from build123d import *

# Parameters (mm, degrees)
EXTRUSION1_DEPTH             = 14
ESQUISSE2_R                  = 3.375
ENL_V_MAT_EXTRU_1_DEPTH      = 11
ENL_V_MAT_EXTRU_2_DEPTH      = 9.5000001
ENL_V_MAT_EXTRU_2_DEPTH_BACK = 9.5000001


with BuildPart() as part:
    # Esquisse1 → Extrusion1 (new body, symmetric)
    with BuildSketch(Plane.XY):
        with BuildLine():
            Line((-8.5, -4.242640687), (-8.5, -3.5))
            ThreePointArc((-8.5, -3.5), (-7.328427125, -0.671572875), (-4.5, 0.5))
            Line((-4.5, 0.5), (4.5, 0.5))
            ThreePointArc((4.5, 0.5), (7.328427125, -0.671572875), (8.5, -3.5))
            Line((8.5, -3.5), (8.5, -4.242640687))
            ThreePointArc((8.5, -4.242640687), (0, -9.5), (-8.5, -4.242640687))
        make_face()
    extrude(amount=EXTRUSION1_DEPTH, both=True)

    # Esquisse2 → Enlèv. mat.-Extru.1 (cut, through all)
    with BuildSketch(Plane(origin=(0, 0.5, 0), x_dir=(-1, 0, 0), z_dir=(0, 1, 0))):
        Circle(ESQUISSE2_R)
    extrude(amount=-ENL_V_MAT_EXTRU_1_DEPTH, mode=Mode.SUBTRACT)

    # Esquisse3 → Enlèv. mat.-Extru.2 (cut, two sides)
    with BuildSketch(Plane(origin=(0, 0, 0), x_dir=(0, 0, -1), z_dir=(1, 0, 0))) as enl_v_mat_extru_2_sk:
        Polygon((14, -9.5), (14, -4.242640687), (9, -9.5), align=None)
        Polygon((-14, -9.5), (-14, -4.242640687), (-9, -9.5), align=None)
    extrude(amount=ENL_V_MAT_EXTRU_2_DEPTH, mode=Mode.SUBTRACT)
    extrude(enl_v_mat_extru_2_sk.sketch, amount=-ENL_V_MAT_EXTRU_2_DEPTH_BACK, mode=Mode.SUBTRACT)


solid = part.part
Read the model definition and answer for the solid it produces. Units are mm, in the model's axes. Coordinates: 2 decimals unless noted, no trailing zeros. Loops run counter-clockwise (first coordinate to the right, second up) from the corner with the lowest first, then second, coordinate; pieces in that order, holes last.
Q1. Consider probe 1 along Z at (x, y) = (0, -2) (3 decimals); probe 2 along X at (y, z) = (-4.25, 0) (3 decimals); probe 3 along Z at (x, y) = (1, -1.5). Determine where each line is inside the solid, lowest interval first.
Q2. The part is cut by section A-A on x = 0. Write down the section's boundary in (y, z) (3 decimals), and give its area (3 significant figures).
Q3. The part is cut by section B-B on z = 0. Write down the section's boundary in (x, y) (3 decimals), and give its area (3 significant figures).
Q4. Each of these flat-tipped pins is pushed along its axis until it touches: pin 1 Ø1 at (y, z) = (-7, 0.5) entering from -X; pin 2 Ø5 at (y, z) = (-8, 4) entering from -X; pin 3 Ø8 at (x, z) = (-6, 0) entering from -Y. Where does it stop, or does it pass through?
Q5. The part is cut by section D-D on z = 9.75. Write down the section's boundary in (x, y).
Q6. The part is cut by section C-C on y = -0.5. Write down the section's boundary in (x, z) (3 decimals).
Q7. The mould has two halves that part along X. Classify faces 1 (the face through (7.297, -0.641, 0.196)), 2 (the face through (0, -2, -14)), 3 (the face through (0.7, -4.4, -3.3)): +X half, -X half, draft (parallel to the pull), parting line (faces both ways), or undercut.
Results below:
1. probe 1: z = -14 to -3.375, 3.375 to 14
1. probe 2: x = -8.496 to -3.375, 3.375 to 8.496
1. probe 3: z = -14 to -3.22, 3.22 to 14
2. outline: (-9.5, -9) - (-4.243, -14) - (0.5, -14) - (0.5, -3.375) - (-9.5, -3.375) - close; (-9.5, 3.375) - (0.5, 3.375) - (0.5, 14) - (-4.243, 14) - (-9.5, 9) - close
2. area: 186 mm2
3. outline: (-8.5, -4.243) arc R9.5 ccw to (-3.375, -8.88) - (-3.375, 0.5) - (-4.5, 0.5) arc R4 ccw to (-8.5, -3.5) - close; (3.375, -8.88) arc R9.5 ccw to (8.5, -4.243) - (8.5, -3.5) arc R4 ccw to (4.5, 0.5) - (3.375, 0.5) - close
3. area: 71.6 mm2
4. pin 1: stops at x = -6.93
4. pin 2: stops at x = -7.75
4. pin 3: stops at y = -9.13
5. outline: (-8.5, -4.24) arc R9.5 ccw to (-3.79, -8.71) - (3.79, -8.71) arc R9.5 ccw to (8.5, -4.24) - (8.5, -3.5) arc R4 ccw to (4.5, 0.5) - (-4.5, 0.5) arc R4 ccw to (-8.5, -3.5) - close
6. outline: (-7.146, -14) - (7.146, -14) - (7.146, 14) - (-7.146, 14) - close; hole circle Ø6.75 at (0, 0)
7. face 1: +X half
7. face 2: draft
7. face 3: undercut
